Geometry check sheet. Reference: drawing and pictorial views, mm from the part's lowest x, y, z. A direction names the side the tool comes from. Coordinates: 2 decimals unless noted, no trailing zeros. Write each loop counter-clockwise with the first axis right and the second up, starting at its lowest first coordinate (ties: lowest second). Pieces come first, ordered by that corner, then holes. Notation, with made-up numbers: (64.5, -21.75) -> (101.5, -21.75) arc R26 cw to (101.5, -1.75) -> close; hole circle Ø4 at (68.5, -7.75). An arc over 180 degrees is marked (long way). Answer in a Markdown table with one row per item.
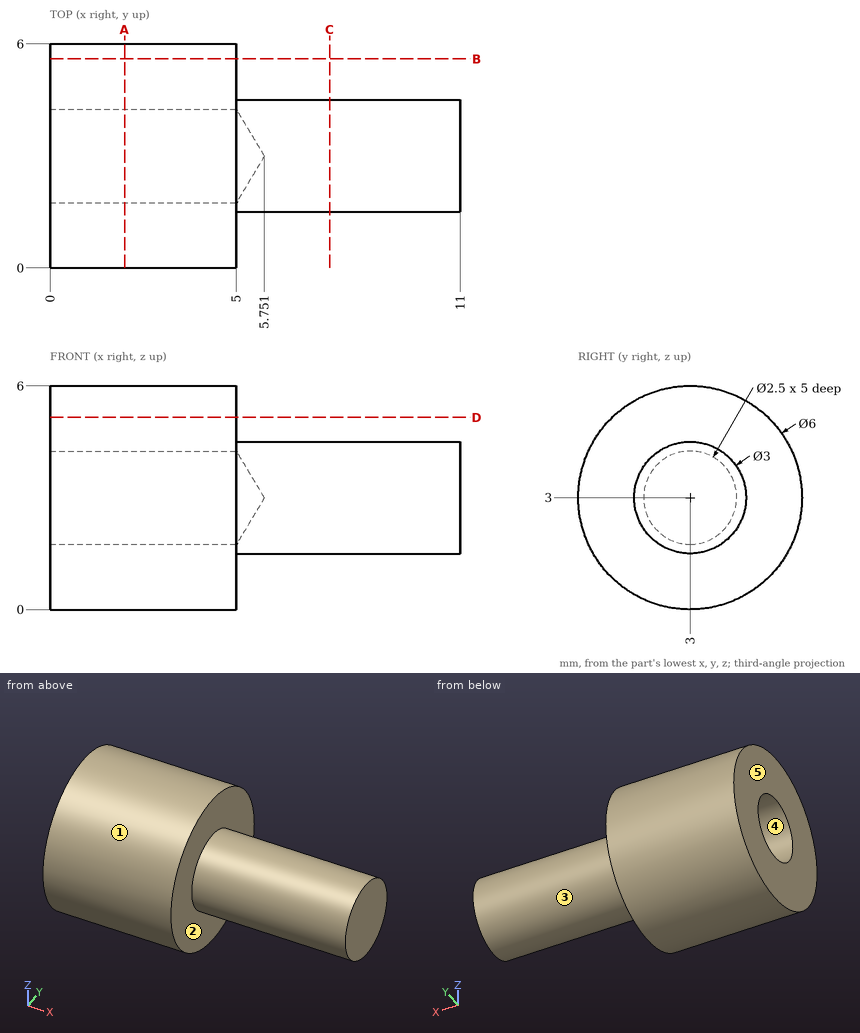
1. Tool access check on the marked faces 1 and 2. Record the directions out of +Z, -Z, +X, -X, +Y, -Y that give a thin tool (end or side, any length) a straight path to the whole face; none if there is none.
Geometry says:
| item | result |
|---|---|
| face 1 | +X, -X |
| face 2 | +X |
2. Section check B-B, the plane y = 5.6. Record the boundary of the cut face in (x, z), plus the area to 3 significant figures.
Geometry says:
| item | result |
|---|---|
| outline | (0, 1.5) -> (5, 1.5) -> (5, 4.5) -> (0, 4.5) -> close |
| area | 15.0 mm^2 |
3. Section check D-D, the plane z = 5.15. Record the boundary of the cut face in (x, y), plus the area to 3 significant figures.
Geometry says:
| item | result |
|---|---|
| outline | (0, 0.91) -> (5, 0.91) -> (5, 5.09) -> (0, 5.09) -> close |
| area | 20.9 mm^2 |
4. Section check A-A, the plane x = 2. Record the boundary of the cut face in (y, z).
Geometry says:
| item | result |
|---|---|
| outline | circle Ø6 at (3, 3); hole circle Ø2.5 at (3, 3) |
5. Thickness scan on line 1 (Z direction, x = 3.85, y = 3); line 2 (X direction, y = 1.45, z = 2.3). Record the ranges inside material, lowest first. Write a range as from..to.
Geometry says:
| item | result |
|---|---|
| line 1 | 0..1.75, 4.25..6 |
| line 2 | 0..5 |
6. Mould release check, pull along Z, two halves, no side actions. Record for the marked faces 3, 4 and 5: released by +Z, released by -Z, zero draft, split by the parting line, or undercut.
Geometry says:
| item | result |
|---|---|
| face 3 | split by the parting line |
| face 4 | undercut |
| face 5 | zero draft |
7. Depth check by flat-ended pin: P1, Ø1.5, axis at x = 5, z = 2, coming from the +Y side. Enter the tip coordinate at first touch or a pass-through.
Geometry says:
| item | result |
|---|---|
| P1 | y = 5.99 |
8. Section check C-C, the plane x = 7.5. Record the boundary of the cut face in (y, z).
Geometry says:
| item | result |
|---|---|
| outline | circle Ø3 at (3, 3) |
